Read the model definition and answer for the solid it produces. Units are mm, in the model's axes. A direction names the side the tool comes from. Coordinates: 2 decimals unless noted, no trailing zeros. Order: outer loops, then holes, each group sorted by start corner. A loop starts at its lowest first (then second) coordinate and runs counter-clockwise, first axis right, second up. Notation, with made-up numbers: (-33, 80.25) - (12, 80.25) arc R24 cw to (12, 107.25) - close; hole circle Ø11 at (-39, 10). An arc over 180 degrees is marked (long way). Write item = value, one per line.
Autodesk Inventor part; units mm, degrees
ref_plane "Work Plane1" through (1.525, 0, 0) normal (0, 0, 1) x (1, 0, 0)
ref_plane "YZ Plane" through (0, 0, 0) normal (1, 0, 0) x (0, 1, 0)
ref_plane "XZ Plane" through (0, 0, 0) normal (0, 1, 0) x (-1, 0, 0)
sketch "Sketch1" plane through (0, 0, 0) normal (0, 0, 1) x (1, 0, 0)
  line L0 (0, 5.7) -> (0, 3.6617)
  line L1 (3.75, 4) -> (35, 4)
  line L2 (35, 4) -> (35, 0)
  line L3 (35, 0) -> (-0.6001, 0)
  line L4 (-7.7201, 0) -> (42.12, 0)
  line L5 (-0.6001, 0) -> (-0.6001, 5.7)
  line L6 (-0.6001, 5.7) -> (0, 5.7)
  line L7 (3.75, 4) -> (2.9831, 3.6617)
  line L8 (2.9831, 3.6617) -> (0, 3.6617)
  line L9 (0, -1.14) -> (0, 6.84)
  dimension "d0" = 35
  dimension "d1" = 31.25
  dimension "d2" = 8
  dimension "d9" = 0.6001
  dimension "d10" = 11.4
  dimension "d13" = 0.7669
  dimension "d14" = 7.3234
revolve "Body" add sketch "Sketch1" angle 360 about axis through (35, 0, 0) along (-1, 0, 0)
sketch "Sketch2" plane through (-0.6001, 0, 0) normal (-1, 0, 0) x (0, 0, 1)
  line L0 (0, 7.5056) -> (6.5, 3.7528)
  line L1 (6.5, 3.7528) -> (6.5, -3.7528)
  line L2 (6.5, -3.7528) -> (0, -7.5056)
  line L3 (0, -7.5056) -> (-6.5, -3.7528)
  line L4 (-6.5, -3.7528) -> (-6.5, 3.7528)
  line L5 (-6.5, 3.7528) -> (0, 7.5056)
  point P0 (0, 0)
  point P1 (0, 0)
  dimension "d11" = 13
extrude "Head" add sketch "Sketch2" along normal blind 4.7
sketch "Sketch4" plane through (0, 0, 0) normal (0, 0, 1) x (1, 0, 0)
  line L0 (-5.3001, 6.5) -> (-5.3001, 7.5056)
  line L1 (-5.3001, 7.5056) -> (-4.7195, 7.5056)
  line L2 (-4.7195, 7.5056) -> (-5.3001, 6.5)
  line L3 (-6.2401, 0) -> (0.3399, 0)
  line L4 (-0.6001, 7.5056) -> (-5.3001, 7.5056)
  line L5 (-5.3001, 3.7528) -> (-5.3001, 7.5056)
  dimension "d5" = 30
  dimension "d19" = 13
revolve "Chamfer1" cut sketch "Sketch4" angle 360 about axis through (-10, 0, 0) along (1, 0, 0)
thread "Thread"
chamfer "Chamfer2" distance 0.7668 distance2 0.7669 1 edges at (35, -4, 0) measured on face at (35, -0.3588, 0.308)
ref_plane "Work Plane1" through (1.525, 0, 0) normal (0, 0, 1) x (1, 0, 0)
equation "\"d0\" = NLG"
equation "\"d1\" = GEL"
equation "\"d2\" = GD"
equation "\"d10\" = SD2"
equation "\"d14\" = BDM"
equation "\"d11\" = SW"
equation "\"d3\" = KOH - SD"
equation "\"d5\" = ANG1"
equation "\"d19\" = SW0"
equation "\"d15\" = GEL"
equation "\"d6\" = -0.5 * SPD + 0.5 * GD"
equation "\"NLG\" = 35"
equation "\"GD\" = NND"
equation "\"BDM\" = 7.32342"
equation "\"KOH\" = 5.3"
equation "\"GEL\" = 31.25"
equation "\"SW\" = 13"
equation "\"SW0\" = 13"
equation "\"SPD\" = NND - 1.2269 * PTC"
equation "\"SD2\" = 11.4"
equation "\"SD\" = 0.6"
equation "\"ANG1\" = 30deg"
equation "\"GAL\" = 0.61345 * PTC"
equation "\"GUL\" = 0.61345 * PTC"
equation "\"RR\" = 0.4"
equation "\"GD1\" = THREADDIA - 1.2269 * PTC"
equation "\"THREADDIA\" = 8"
equation "\"TOA\" = 30deg"
equation "\"PTC\" = 1.25"
equation "\"NND\" = 8"
equation "\"E0\" = 1.155 * SW"
properties part number "DIN 933 - M8  x 35" material "Steel, Mild"
1) The part is cut by section B-B (x = 20). Determine the outline of the cut face in (y, z), and give its area (3 significant figures).
Returned:
outline = circle Ø8 at (0, 0)
area = 50.3 mm^2
2) Determine the mould class of faces 1 (the face through (-0.6, -6, -1)), 2 (the face through (1.47, -3.66, -0.16)), 3 (the face through (-2.92, -5.66, -3.2)) for opening direction X: pulls with the +X half, pulls with the -X half, needs draft (parallel to the pull), parting line crosses it, or undercut.
Returned:
face_1 = pulls with the +X half
face_2 = undercut
face_3 = needs draft
3) Flat-ended cylindrical pins translate along their axes: pin 1 Ø3 at (x, y) = (7, -4.5) entering from +Z; pin 2 Ø1.5 at (x, z) = (22, 2) entering from -Y; pin 3 Ø1 at (x, z) = (13, 1) entering from -Y. Find the tip coordinate at first contact, or state that the pin passes through.
Returned:
pin_1 = 2.65
pin_2 = -3.8
pin_3 = -3.97
4) Straight lines are drawn through the part: line 1 along X through (y, z) = (6.25, -0.5); line 2 along X through (y, z) = (-3, 2.25); line 3 along X through (y, z) = (5.5, 0). For each, find the intervals that lie inside material, in ascending order. Write a range as from..to.
Returned:
line_1 = -5.3..-0.6
line_2 = -5.3..0, 3.18..34.48
line_3 = -5.3..0
5) For faces 4 (the face through (0, 0, 4)), 5 (the face through (-3, 0, -6.5)), 6 (the face through (19.205, -0.867, -3.905)), determine the directions among +Z, -Z, +X, -X, +Y, -Y from which every point of the face is accessible in a straight line to the end or side of a thin tool.
Returned:
face_4 = none
face_5 = -Z, +X, -X, +Y, -Y
face_6 = +X
6) The part is cut by section A-A (x = -1). Determine the outline of the cut face in (y, z).
Returned:
outline = (-7.51, 0) - (-3.75, -6.5) - (3.75, -6.5) - (7.51, 0) - (3.75, 6.5) - (-3.75, 6.5) - close
